Read the model definition and answer for the solid it produces. Units are mm, in the model's axes. A direction names the side the tool comes from. Coordinates: 2 decimals unless noted, no trailing zeros. Loops run counter-clockwise (first coordinate to the right, second up) from the corner with the lowest first, then second, coordinate; pieces in that order, holes last.
from build123d import *

# Parameters (mm, degrees)
CUT_EXTRUDE1_START = 8.5
CUT_EXTRUDE1_DEPTH = 1.5


with BuildPart() as part:
    # Sketch2 → Revolve1 (revolve)
    with BuildSketch(Plane(origin=(0, 0, 0), x_dir=(0, 0, -1), z_dir=(1, 0, 0)), mode=Mode.PRIVATE) as revolve1_sk:
        with BuildLine():
            Line((8.5, 0), (8.5, 1))
            Line((8.5, 1), (8, 1.5))
            Line((8, 1.5), (-5.5, 1.5))
            Line((-5.5, 1.5), (-5.5, 2.6))
            ThreePointArc((-5.5, 2.6), (-5.543933983, 2.706066017), (-5.65, 2.75))
            Line((-5.65, 2.75), (-8.35, 2.75))
            ThreePointArc((-8.35, 2.75), (-8.456066017, 2.706066017), (-8.5, 2.6))
            Line((-8.5, 2.6), (-8.5, 0))
            Line((-8.5, 0), (8.5, 0))
        make_face()
    revolve(revolve1_sk.sketch.rotate(Axis((0, 0, -8.5), (0, 0, 1)), 90), axis=Axis((0, 0, -8.5), (0, 0, 1)))

    # Sketch3 → Cut-Extrude1 (cut)
    with BuildSketch(Plane.XY.offset(CUT_EXTRUDE1_START)):
        Polygon((-1.25, 0.721687836), (-1.25, -0.721687836), (0, -1.443375673), (1.25, -0.721687836), (1.25, 0.721687836), (0, 1.443375673), align=None)
    extrude(amount=-CUT_EXTRUDE1_DEPTH, mode=Mode.SUBTRACT)

    # Cut-Extrude2 cone 1 section (through the dimple's axis) → Cut-Extrude2 (revolve, cut)
    with BuildSketch(Plane(origin=(0, 0, 8.5), x_dir=(0, -1, 0), z_dir=(1, 0, 0))):
        Polygon((0, 0), (1.636146394, 0), (0, 0.944629561), align=None)
    revolve(axis=Axis((0, 0, 8.5), (0, 0, -1)), mode=Mode.SUBTRACT)


solid = part.part
Q1. A cutting plane is placed at A-A (y = 0). Give the vertices of the cut face in (x, z).
Findings below:
outline: (-2.75, 5.65) arc R0.15 ccw to (-2.6, 5.5) - (-1.5, 5.5) - (-1.5, -8) - (-1, -8.5) - (1, -8.5) - (1.5, -8) - (1.5, 5.5) - (2.6, 5.5) arc R0.15 ccw to (2.75, 5.65) - (2.75, 8.35) arc R0.15 ccw to (2.6, 8.5) - (1.64, 8.5) - (1.25, 8.28) - (1.25, 7) - (-1.25, 7) - (-1.25, 8.28) - (-1.64, 8.5) - (-2.6, 8.5) arc R0.15 ccw to (-2.75, 8.35) - close
Q2. Determine the mould class of faces 4 (the face through (0, 2, 8.5)), 5 (the face through (0.63, 1.08, 7.7)), 6 (the face through (0, 0, 7)), 7 (the face through (0.596, 2.685, 7.019)) for opening direction X: +X half, -X half, draft (parallel to the pull), parting line (faces both ways), or undercut.
Findings below:
face 4: draft
face 5: undercut
face 6: undercut
face 7: parting line
Q3. A cutting plane is placed at C-C (z = 6.5). Give the vertices of the cut face in (x, y).
Findings below:
outline: circle Ø5.5 at (0, 0)
Q4. Straight lines are drawn through the part: probe 1 along Z at (x, y) = (1, 1.4); probe 2 along Y at (x, z) = (-0.05, 7.75); probe 3 along Y at (x, z) = (-1.2, 7.25). For each, find the intervals that lie inside material, in ascending order.
Findings below:
probe 1: z = 5.5 to 8.5
probe 2: y = -2.75 to -1.41, 1.41 to 2.75
probe 3: y = -2.47 to -0.75, 0.75 to 2.47
Q5. Which of the six approach directions +Z, -Z, +X, -X, +Y, -Y give full straight-line access (tool end or side, diameter ignored) to faces 1 (the face through (1.25, 0, 8)), 2 (the face through (0, 2, 5.5)), 3 (the face through (0, 0, -8.5))?
Findings below:
face 1: +Z
face 2: -Z
face 3: -Z, +X, -X, +Y, -Y
Q6. A cutting plane is placed at B-B (z = -6.75). Give the vertices of the cut face in (x, y), then the cut area to 3 significant figures.
Findings below:
outline: circle Ø3 at (0, 0)
area: 7.07 mm2
Q7. Flat-ended cylindrical pins translate along their axes: pin 1 Ø2 at (x, y) = (-1.5, 1.5) entering from -Z; pin 2 Ø1.2 at (x, y) = (0, -0.5) entering from +Z; pin 3 Ø1.5 at (y, z) = (0, -5) entering from +X. Find the tip coordinate at first contact, or state that the pin passes through.
Findings below:
pin 1: stops at z = -8.38
pin 2: stops at z = 7
pin 3: stops at x = 1.5
